```python
from build123d import *

# Parameters (mm, degrees)
SKETCH_1_R               = 82.5
EXTRUDE_1_DEPTH          = 70
EXTRUDE_START            = -407.460947
SKETCH_2_R               = 20
EXTRUDE_2_DEPTH          = 407.460947
EXTRUDE_START_2          = -489.960947
SKETCH_4_R               = 20
EXTRUDE_3_DEPTH          = 489.960947
PATTERN_CIRCULAR_2_COUNT = 2


with BuildPart() as part:
    # 스케치1 → 보스-돌출1 (new body)
    with BuildSketch(Plane(origin=(0, 0, 0), x_dir=(1, 0, 0), z_dir=(0, 1, 0))):
        with Locations(Location((0, 0, 0), (0, 0, 270))):  # turned: the seam where the file's is
            Circle(SKETCH_1_R)
        with BuildLine():
            Line((61.694813396, -10), (67, -10))
            Line((67, -10), (67, 10))
            Line((67, 10), (61.694813396, 10))
            ThreePointArc((61.694813396, 10), (-62.5, 0), (61.694813396, -10))
        make_face(mode=Mode.SUBTRACT)
    extrude(amount=EXTRUDE_1_DEPTH)

    # 스케치2 → 보스-돌출2 (add)
    with BuildSketch(Plane.XY.offset(487.5).offset(EXTRUDE_START)):
        with Locations((0, 35)):
            Circle(SKETCH_2_R)
    extrude_2 = extrude(amount=EXTRUDE_2_DEPTH)

    # 스케치4 → 보스-돌출3 (add)
    with BuildSketch(Plane(origin=(570, 0, 0), x_dir=(0, 0, -1), z_dir=(1, 0, 0)).offset(EXTRUDE_START_2)):
        with Locations((0, 35)):
            Circle(SKETCH_4_R)
    extrude_3 = extrude(amount=EXTRUDE_3_DEPTH)

    # 원형 패턴2: 보스-돌출2, 보스-돌출3 ×2 about axis
    pattern_circular_2_axis = Axis((0, 0, 0), (0, 1, 0))
    add([extrude_2.rotate(pattern_circular_2_axis, i * 360 / PATTERN_CIRCULAR_2_COUNT) for i in range(1, PATTERN_CIRCULAR_2_COUNT)])
    add([extrude_3.rotate(pattern_circular_2_axis, i * 360 / PATTERN_CIRCULAR_2_COUNT) for i in range(1, PATTERN_CIRCULAR_2_COUNT)])


solid = part.part
```
Could you check a few things on this model? Use its own coordinates, in mm. A direction names the side the tool comes from. Give positions to 0.01 mm unless a question says otherwise; leave off trailing zeros. Loops run counter-clockwise (first coordinate to the right, second up) from the corner with the lowest first, then second, coordinate; pieces in that order, holes last. Notation, with made-up numbers: (-26, 45.25) -> (28, 45.25) arc R33 cw to (28, 73.25) -> close; hole circle Ø2 at (79, 88.5). An arc over 180 degrees is marked (long way). Put each result on its own line as item: value.
(1) Imagine slicing it at D-D on z = 119. Write out the boundary of the cut face in (x, y), plus the area to 3 significant figures.
Computed:
outline: circle Ø40 at (0, 35)
area: 1,260 mm^2
(2) Thinking about a two-plate mould opening in X: for faces 6 (the face through (-2.6, 54.83, 280.92)), 7 (the face through (61.5, 0, -12.6)), 8 (the face through (-62.446, 34.51, -2.608)), which applies, pulls with the +X half, pulls with the -X half, needs draft (parallel to the pull), parting line crosses it, or undercut?
Computed:
face 6: parting line crosses it
face 7: needs draft
face 8: undercut
(3) For faces 1 (the face through (321.59, 54.83, 2.6)), 2 (the face through (2.6, 54.83, -280.92)), 3 (the face through (61.5, 70, -12.6)), 4 (the face through (0, 35, 487.5)), 5 (the face through (-321.59, 54.83, -2.6)), which set-ups out of +Z, -Z, +X, -X, +Y, -Y let a thin tool reach every point of the face, with its end or its side?
Computed:
face 1: +X
face 2: -Z
face 3: +Z, -Z, +X, -X, +Y
face 4: +Z, +X, -X, +Y, -Y
face 5: -X
(4) Please list where these lines run through material, in increasing order: probe 1 along X at (y, z) = (54.5, 0); probe 2 along Z at (x, y) = (0, 25); probe 3 along X at (y, z) = (35.5, 360.5). Write a range as [from, to].
Computed:
probe 1: [-570, -62.5], [67, 570]
probe 2: [-487.5, -62.5], [62.5, 487.5]
probe 3: [-19.99, 19.99]
(5) Imagine slicing it at B-B on x = 0. Write out the boundary of the cut face in (y, z).
Computed:
outline: (0, -82.5) -> (15, -82.5) -> (15, -487.5) -> (55, -487.5) -> (55, -82.5) -> (70, -82.5) -> (70, -62.5) -> (0, -62.5) -> close; (0, 62.5) -> (70, 62.5) -> (70, 82.5) -> (55, 82.5) -> (55, 487.5) -> (15, 487.5) -> (15, 82.5) -> (0, 82.5) -> close
(6) Imagine slicing it at A-A on y = 35. Write out the boundary of the cut face in (x, z).
Computed:
outline: (-570, -20) -> (-80.04, -20) arc R82.5 ccw to (-20, -80.04) -> (-20, -487.5) -> (20, -487.5) -> (20, -80.04) arc R82.5 ccw to (80.04, -20) -> (570, -20) -> (570, 20) -> (80.04, 20) arc R82.5 ccw to (20, 80.04) -> (20, 487.5) -> (-20, 487.5) -> (-20, 80.04) arc R82.5 ccw to (-80.04, 20) -> (-570, 20) -> close; hole (61.69, -10) -> (67, -10) -> (67, 10) -> (61.69, 10) arc R62.5 ccw (long way) to start
(7) I'm going to push flat-ended pins straight in: pin 1 Ø1 at (x, y) = (48, 34.5) entering from +Z; pin 2 Ø1.6 at (x, y) = (64.5, 51) entering from +Z; pin 3 Ø1.5 at (x, y) = (-224.5, 45) entering from -Z. Where does each tip first touch, or does it pass through?
Computed:
pin 1: z = 67.45
pin 2: z = 52.43
pin 3: z = -17.73
(8) Imagine slicing it at C-C on x = 195.5. Write out the boundary of the cut face in (y, z).
Computed:
outline: circle Ø40 at (35, 0)
